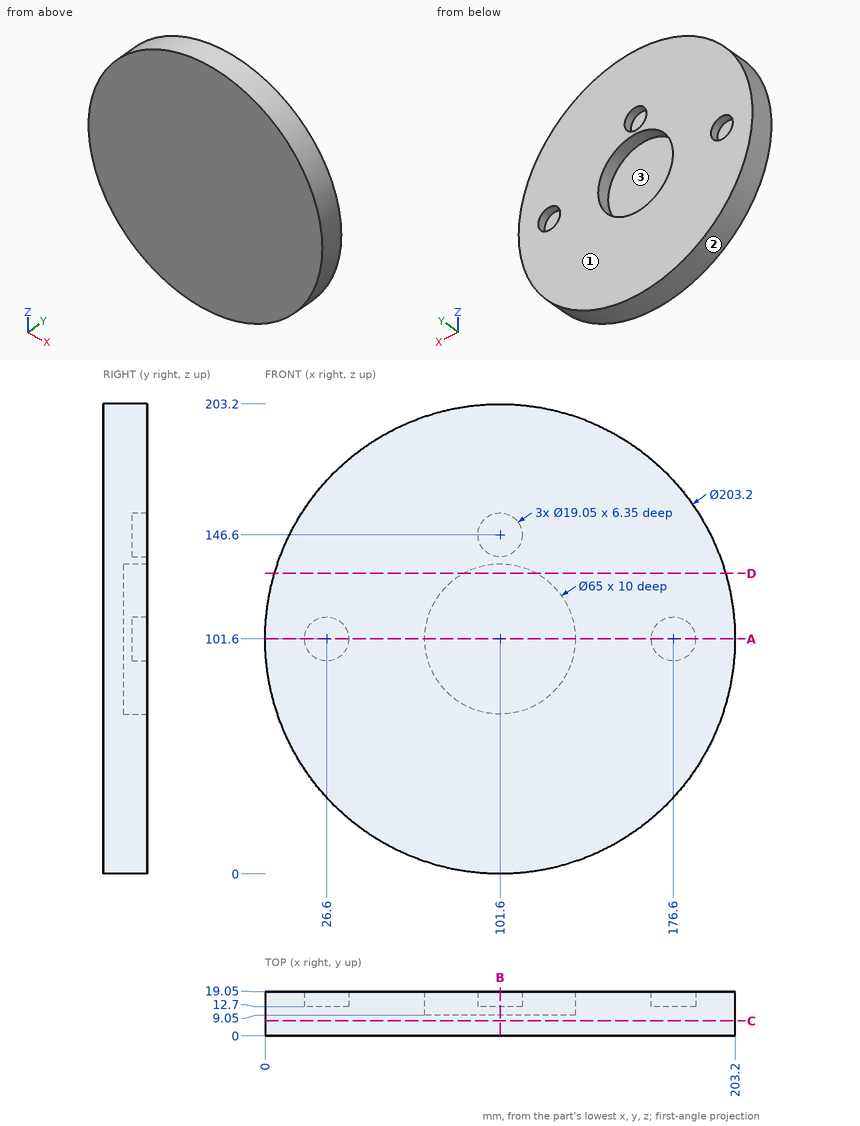
Part print with two shaded views. Sizes in mm from the minimum x, y, z corner. Round coordinates to 2 decimals unless told otherwise and drop trailing zeros. Order: outer loops, then holes, each group sorted by start corner. A loop starts at its lowest first (then second) coordinate and runs counter-clockwise, first axis right, second up. Notation, with made-up numbers: M 21.5,-4.75 L 30.5,-4.75 A13 ccw 30.5,-0.75 Z; hole C -24,42 d8. An arc over 180 degrees is marked long. Use CSV: the item, a comma, the result in double quotes. Start each with the question number.
(1) Cut at B-B on x = 101.6. List the corners of the cut face in (y, z) (3 decimals).
(2) Drill centre lines: probe 1 along Z at (x, y) = (102, 16.5); probe 2 along X at (y, z) = (17, 101.6) (3 decimals); probe 3 along Z at (x, y) = (26.6, 17.5) (3 decimals). Where is each one in solid material? Low to high.
(3) Mould opens along Z. For the marked faces 1, 2 and 3 say: +Z half, -Z half, draft (parallel to the pull), parting line (faces both ways), or undercut.
(4) Cut at C-C on y = 6.5. List the corners of the cut face in (x, z).
(5) Cut at A-A on z = 101.6. List the corners of the cut face in (x, y) (3 decimals), then the cut area to 3 significant figures.
(6) Cut at D-D on z = 130. List the corners of the cut face in (x, y), then the cut area to 3 significant figures.
(7) Flat gauge pins, fed straight in: P1, Ø9.5, axis at x = 173.5, z = 100, coming from the +Y side; P2, Ø1.5, axis at x = 127.5, z = 151, coming from the -Y side; P3, Ø2, axis at y = 17, z = 107, coming from the -X side; P4, Ø10, axis at y = 15, z = 136.5, coming from the +X side. Where does each tip first touch, or does it go through?
Findings:
1,outline,"M 0,0 L 19.05,0 L 19.05,69.1 L 9.05,69.1 L 9.05,134.1 L 19.05,134.1 L 19.05,137.075 L 12.7,137.075 L 12.7,156.125 L 19.05,156.125 L 19.05,203.2 L 0,203.2 Z"
2,probe 1,"z = 0 to 69.1, 134.1 to 137.08, 156.12 to 203.2"
2,probe 2,"x = 0 to 17.075, 36.125 to 69.1, 134.1 to 167.075, 186.125 to 203.2"
2,probe 3,"z = 33.061 to 92.075, 111.125 to 170.139"
3,face 1,"draft"
3,face 2,"parting line"
3,face 3,"undercut"
4,outline,"C 101.6,101.6 d203.2"
5,outline,"M 0,0 L 203.2,0 L 203.2,19.05 L 186.125,19.05 L 186.125,12.7 L 167.075,12.7 L 167.075,19.05 L 134.1,19.05 L 134.1,9.05 L 69.1,9.05 L 69.1,19.05 L 36.125,19.05 L 36.125,12.7 L 17.075,12.7 L 17.075,19.05 L 0,19.05 Z"
5,area,"2,980 mm^2"
6,outline,"M 4.05,0 L 199.15,0 L 199.15,19.05 L 117.4,19.05 L 117.4,9.05 L 85.8,9.05 L 85.8,19.05 L 4.05,19.05 Z"
6,area,"3,400 mm^2"
7,P1,"stops at y = 12.7"
7,P2,"stops at y = 0"
7,P3,"stops at x = 0.1"
7,P4,"stops at x = 198.7"
